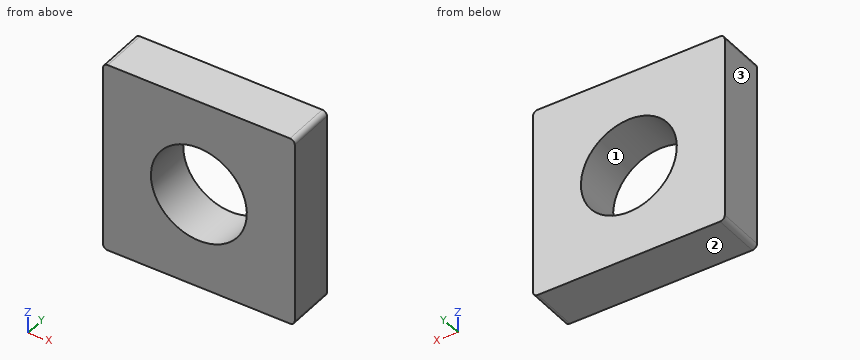
```python
from build123d import *

# Parameters (mm, degrees)
SKETCH_1_W      = 8
SKETCH_1_H      = 8
SKETCH_1_R      = 2
EXTRUDE_1_DEPTH = 1
FILLET_1_R      = 0.2


with BuildPart() as part:
    # 草图1 → 凸台-拉伸1 (new, symmetric)
    with BuildSketch(Plane(origin=(0, 0, 0), x_dir=(1, 0, 0), z_dir=(0, 1, 0))):
        Rectangle(SKETCH_1_W, SKETCH_1_H)
        with Locations(Location((0, 0, 0), (0, 0, 270))):
            Circle(SKETCH_1_R, mode=Mode.SUBTRACT)
    extrude(amount=EXTRUDE_1_DEPTH, both=True)

    # 圆角1
    fillet_1_edges = [part.edges().sort_by_distance(p)[0] for p in [
        (4, 0, 4),
        (-4, 0, 4),
        (-4, 0, -4),
        (4, 0, -4),
    ]]
    fillet(fillet_1_edges, radius=FILLET_1_R)


solid = part.part
```
Work out the finished part from the listing and answer in its coordinate system (mm). Face numbers are marked on the shaded views. Round coordinates to 2 decimals unless told otherwise and drop trailing zeros. Write each loop counter-clockwise with the first axis right and the second up, starting at its lowest first coordinate (ties: lowest second). Pieces come first, ordered by that corner, then holes. Notation, with made-up numbers: (43, -39) - (84, -39) arc R23 ccw to (84, -1) - close; hole circle Ø4 at (-0.75, 16). An arc over 180 degrees is marked (long way). Return JSON: item names as keys, results as strings. Group by question number.
Q1. The part is cut by section A-A on x = 0. Write down the section's boundary in (y, z).
Q2. Find the intervals of material crossed by L1, parallel to X at y = -0.05, z = 0; L2, parallel to X at y = 0.65, z = 1.75; L3, parallel to Z at x = 0.25, y = -0.7, in increasing order.
Q3. The part is cut by section C-C on z = 0. Write down the section's boundary in (x, y), then the cut area to 3 significant figures.
Q4. This flat-tipped pin is pushed along its axis until it touches: pin 1 Ø4 at (x, z) = (-1, -1) entering from -Y. Where does it stop, or does it pass through?
Q5. The part is cut by section B-B on y = -0.75. Write down the section's boundary in (x, z).
Q6. The mould has two halves that part along X. Classify the marked faces 1, 2 and 3: released by +X, released by -X, zero draft, split by the parting line, or undercut.
Solved:
{
 "1": {"outline": "(-1, -4) - (1, -4) - (1, -2) - (-1, -2) - close; (-1, 2) - (1, 2) - (1, 4) - (-1, 4) - close"},
 "2": {"L1": "-4 to -2, 2 to 4", "L2": "-4 to -0.97, 0.97 to 4", "L3": "-4 to -1.98, 1.98 to 4"},
 "3": {"outline": "(-4, -1) - (-2, -1) - (-2, 1) - (-4, 1) - close; (2, -1) - (4, -1) - (4, 1) - (2, 1) - close", "area": "8.00 mm²"},
 "4": {"pin 1": "y = -1"},
 "5": {"outline": "(-4, -3.8) arc R0.2 ccw to (-3.8, -4) - (3.8, -4) arc R0.2 ccw to (4, -3.8) - (4, 3.8) arc R0.2 ccw to (3.8, 4) - (-3.8, 4) arc R0.2 ccw to (-4, 3.8) - close; hole circle Ø4 at (0, 0)"},
 "6": {"face 1": "undercut", "face 2": "zero draft", "face 3": "released by -X"}
}
